Work out the finished part from the listing and answer in its coordinate system (mm). A direction names the side the tool comes from. Give positions to 0.01 mm unless a question says otherwise; leave off trailing zeros. Use a Markdown table: item, result. Add a question column.
Q1. For faces 1 (the face through (572.212, 299.865, 7.465)), 2 (the face through (619, 441, 10)), determine the directions among +Z, -Z, +X, -X, +Y, -Y from which every point of the face is accessible in a straight line to the end or side of a thin tool.
Q2. Consider line 1 (Y direction, x = 560, z = 7); line 2 (X direction, y = 125, z = 5.25); line 3 (X direction, y = 704, z = 7.5). Determine where each line is inside the solid, lowest interval first.
Q3. For a pull along X with two mould halves and no side action, classify faces 3 (the face through (325, 441, 0)), 4 (the face through (178.946, 136.464, 7.465)), 5 (the face through (553.116, 269.366, 7.465)) as pulls with the +X half, pulls with the -X half, needs draft (parallel to the pull), parting line crosses it, or undercut.
from build123d import *

# Parameters (mm, degrees)
ESQUISSE1_W             = 660
ESQUISSE1_H             = 870
BOSS_EXTRU_1_DEPTH      = 10
ENL_V_MAT_EXTRU_1_DEPTH = 5
CHANFREIN1_SIZE         = 5


with BuildPart() as part:
    # Esquisse1 → Boss.-Extru.1 (new body)
    with BuildSketch(Plane.XY):
        with Locations((330, 435)):
            Rectangle(ESQUISSE1_W, ESQUISSE1_H)
    extrude(amount=BOSS_EXTRU_1_DEPTH)

    # Esquisse2 → Enlèv. mat.-Extru.1 (cut)
    with BuildSketch(Plane.XY.offset(10)):
        Polygon((120, 328.492424049), (120, 541.507575951), (60, 601.507575951), (60, 268.492424049), align=None)
        Polygon((268.492424049, 690), (391.507575951, 690), (511.507575951, 810), (148.492424049, 810), align=None)
        Polygon((60, 810), (60, 643.933982822), (150, 553.933982822), (150, 316.066017178), (60, 226.066017178), (60, 60), (106.066017178, 60), (256.066017178, 210), (403.933982822, 210), (553.933982822, 60), (600, 60), (600, 226.066017178), (510, 316.066017178), (510, 553.933982822), (600, 643.933982822), (600, 810), (553.933982822, 810), (403.933982822, 660), (256.066017178, 660), (106.066017178, 810), align=None)
        Polygon((540, 328.492424049), (540, 541.507575951), (600, 601.507575951), (600, 268.492424049), align=None)
        Polygon((511.507575951, 60), (148.492424049, 60), (268.492424049, 180), (391.507575951, 180), align=None)
    extrude(amount=-ENL_V_MAT_EXTRU_1_DEPTH, mode=Mode.SUBTRACT)

    # Chanfrein1
    chanfrein1_edges = [part.edges().sort_by_distance(p)[0] for p in [
        (330, 60, 5),
        (208.492424049, 120, 5),
        (330, 180, 5),
        (451.507575951, 120, 5),
        (60, 435, 5),
        (90, 571.507575951, 5),
        (120, 435, 5),
        (90, 298.492424049, 5),
        (600, 435, 5),
        (570, 298.492424049, 5),
        (540, 435, 5),
        (570, 571.507575951, 5),
        (181.066017178, 735, 5),
        (330, 660, 5),
        (478.933982822, 735, 5),
        (576.966991411, 810, 5),
        (600, 726.966991411, 5),
        (555, 598.933982822, 5),
        (510, 435, 5),
        (555, 271.066017178, 5),
        (600, 143.033008589, 5),
        (576.966991411, 60, 5),
        (478.933982822, 135, 5),
        (330, 210, 5),
        (181.066017178, 135, 5),
        (83.033008589, 60, 5),
        (60, 143.033008589, 5),
        (105, 271.066017178, 5),
        (150, 435, 5),
        (105, 598.933982822, 5),
        (60, 726.966991411, 5),
        (83.033008589, 810, 5),
        (330, 810, 5),
        (451.507575951, 750, 5),
        (330, 690, 5),
        (208.492424049, 750, 5),
    ]]
    chamfer(chanfrein1_edges, length=CHANFREIN1_SIZE - 0.0001)  # a hair under: the kernel refuses the full size


solid = part.part
Result set:
| question | item | result |
|---|---|---|
| 1 | face 1 | +Z |
| 1 | face 2 | +Z, +X, -X, +Y, -Y |
| 2 | line 1 | y = 0 to 63, 261.82 to 312.73, 557.27 to 608.18, 807 to 870 |
| 2 | line 2 | x = 0 to 64.75, 164.35 to 220.21, 439.79 to 495.65, 595.25 to 660 |
| 2 | line 3 | x = 0 to 62.5, 208.53 to 258.03, 401.97 to 451.47, 597.5 to 660 |
| 3 | face 3 | needs draft |
| 3 | face 4 | undercut |
| 3 | face 5 | undercut |
